Source: CAD feature listing. Evaluate the final solid. Frame: model axes, mm. Face numbers are marked on the shaded views. A direction names the side the tool comes from. Give positions to 0.01 mm unless a question says otherwise; leave off trailing zeros. Loops run counter-clockwise (first coordinate to the right, second up) from the corner with the lowest first, then second, coordinate; pieces in that order, holes last. Notation, with made-up numbers: (79, 1) -> (126, 1) arc R29 ccw to (126, 24) -> close; hole circle Ø2 at (33, 26.25). An arc over 180 degrees is marked (long way). Return JSON: item names as keys, results as strings. Group by question number.
(1) Pin query (flat end, axial travel): pin 1 (4 mm diameter, centred on x = 22.5, y = 47.5, fed in from -Z); pin 2 (3.5 mm diameter, centred on x = 8.5, y = -31.5, fed in from -Z); pin 3 (3 mm diameter, centred on y = 15.5, z = 10.5, fed in from +X); pin 4 (1.5 mm diameter, centred on x = -17, z = 6, fed in from +Y). Return the tip coordinate at first contact, or that it passes through.
(2) Ray query, line 1 (X direction, y = -28, z = 16.5); line 2 (Y direction, x = 0, z = 6.25); line 3 (Y direction, x = 12, z = 17.75). Return the intervals inside material, ascending. Write a range as from..to.
(3) Access query for the marked faces 1, 2 and 3. Directions: +Z, -Z, +X, -X, +Y, -Y. A direction counts if a zero-diameter tool reaches every point of the face in a straight line with its end or side. Return the directions, or none.
(4) Cut plane C-C on z = 6.5. Return loops of the section in (x, y).
(5) Draft query along Y for the marked faces 4, 5, 6 and 7. Return one class per face: released by +Y, released by -Y, zero draft, split by the parting line, or undercut.
(6) Cut plane B-B on y = 3.5. Return loops of the section in (x, z), then the cut area to 3 significant figures.
(7) Cut plane A-A on x = 0. Return loops of the section in (y, z).
(8) Cut plane D-D on x = -12. Give the number of separate pieces and of enclosed holes in the cut face, then the cut area to 3 significant figures.
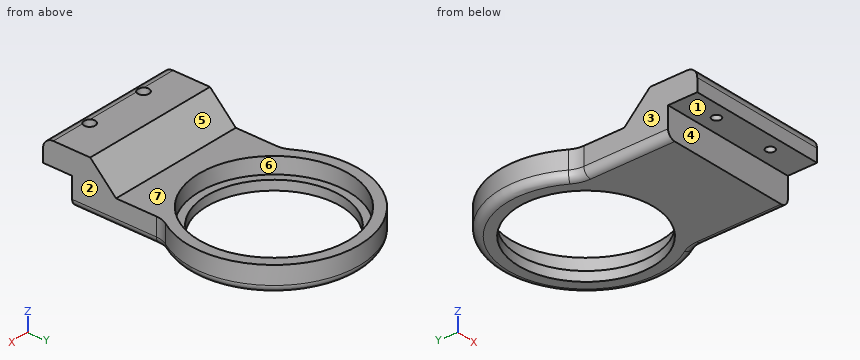
```python
from build123d import *

# Parameters (mm, degrees)
SKETCH_1_R          = 26
EXTRUDE_1_DEPTH     = 10
SKETCH_3_R          = 29
CUT_EXTRUDE_1_DEPTH = 6.3
FILLET_1_R          = 9
SKETCH_4_W          = 53.328443722
SKETCH_4_H          = 11.316007496
EXTRUDE_2_DEPTH     = 10
SKETCH_5_W          = 53.328443722
SKETCH_5_H          = 11.316007496
EXTRUDE_3_DEPTH     = 2
SKETCH_6_W          = 53.328443722
SKETCH_6_H          = 10
EXTRUDE_4_DEPTH     = 3
CHAMFER_1_SIZE      = 14
FILLET_3_R          = 3
SKETCH_7_R          = 1.7
CUT_EXTRUDE_2_DEPTH = 14
SKETCH_8_R          = 2.15
SKETCH_8_R_2        = 2.165
CUT_EXTRUDE_3_DEPTH = 6
SKETCH_9_W          = 53.328443722
SKETCH_9_H          = 11.316007496
CUT_EXTRUDE_4_DEPTH = 3
FILLET_4_R          = 4


with BuildPart() as part:
    # Sketch 1 → Extrude 1 (new body)
    with BuildSketch(Plane.XY):
        with BuildLine():
            Line((26.664221861, -27.841996252), (-26.664221861, -27.841996252))
            Line((-26.664221861, -27.841996252), (-26.664221861, 7.574088737))
            ThreePointArc((-26.664221861, 7.574088737), (0, 60.241390131), (26.664221861, 7.574088737))
            Line((26.664221861, 7.574088737), (26.664221861, -27.841996252))
        make_face()
        with Locations((0, 27.158003748)):
            Circle(SKETCH_1_R, mode=Mode.SUBTRACT)
    extrude(amount=EXTRUDE_1_DEPTH)

    # Sketch 3 → Cut-Extrude 1 (cut)
    with BuildSketch(Plane.XY.offset(10)):
        with Locations((0, 27.158003748)):
            Circle(SKETCH_3_R)
    extrude(amount=-CUT_EXTRUDE_1_DEPTH, mode=Mode.SUBTRACT)

    # Fillet 1
    fillet_1_edges = [part.edges().sort_by_distance(p)[0] for p in [
        (-26.664221861, 7.574088737, 5),
        (26.664221861, 7.574088737, 5),
    ]]
    fillet(fillet_1_edges, radius=FILLET_1_R)



with BuildPart() as body_2:
    # Sketch 4 → Extrude 2 (new body)
    with BuildSketch(Plane.XY.offset(10)):
        with Locations((0, -33.5)):
            Rectangle(SKETCH_4_W, SKETCH_4_H)
    extrude(amount=EXTRUDE_2_DEPTH)


with BuildPart() as part_1:
    add(part.part)

    add(body_2.part)  # Extrude 3 merges body 2
    # Sketch 5 → Extrude 3 (add)
    with BuildSketch(Plane(origin=(0, 0, 10), x_dir=(-1, 0, 0), z_dir=(0, 0, -1))):
        with Locations((0, -33.5)):
            Rectangle(SKETCH_5_W, SKETCH_5_H)
    extrude(amount=EXTRUDE_3_DEPTH)

    # Sketch 6 → Extrude 4 (add)
    with BuildSketch(Plane(origin=(0, -27.841996252, 0), x_dir=(1, 0, 0), z_dir=(0, 1, 0))):
        with Locations((0, -15)):
            Rectangle(SKETCH_6_W, SKETCH_6_H)
    extrude(amount=EXTRUDE_4_DEPTH)

    # Chamfer 1
    # the kernel refuses this chamfer: 14 mm, written as the material it adds along each edge
    with BuildSketch(Plane(origin=(-26.664221861, -24.841996252, 10), x_dir=(0, -0.027495876610586365, 0.9996219169112968), z_dir=(1, 0, 0))) as chamfer_1_piece_1_section:
        Polygon((CHAMFER_1_SIZE * 0.999621916911, -CHAMFER_1_SIZE * 0.0274958766106), (-CHAMFER_1_SIZE * 0.0274958766106, -CHAMFER_1_SIZE * 0.999621916911), (0, 0), align=None)
    chamfer_1_piece_1 = extrude(amount=53.328443723, mode=Mode.PRIVATE)
    chamfer_1_piece_1 = split(chamfer_1_piece_1, bisect_by=Plane(origin=(0, -19.845516644, 20), z_dir=(0, 0, -1)), keep=Keep.TOP, mode=Mode.PRIVATE)
    add(chamfer_1_piece_1)

    # Fillet 3
    fillet_3_edges = [part_1.edges().sort_by_distance(p)[0] for p in [
        (-26.664221861, -11.511986052, 0),
        (0, 60.241390131, 0),
        (-27.014230163, 7.303510743, 0),
        (27.014230163, 7.303510743, 0),
        (26.664221861, -11.511986052, 0),
    ]]
    fillet(fillet_3_edges, radius=FILLET_3_R)

    # Sketch 7 → Cut-Extrude 2 (cut)
    with BuildSketch(Plane(origin=(0, 0, 8), x_dir=(-1, 0, 0), z_dir=(0, 0, -1))):
        with Locations((-12, -33.841996252)):
            Circle(SKETCH_7_R)
        with Locations((12, -33.841996252)):
            Circle(SKETCH_7_R)
    extrude(amount=-CUT_EXTRUDE_2_DEPTH, mode=Mode.SUBTRACT)

    # Sketch 8 → Cut-Extrude 3 (cut)
    with BuildSketch(Plane.XY.offset(20)):
        with Locations((-12, -33.841996252)):
            Circle(SKETCH_8_R)
        with Locations((12, -33.841996252)):
            Circle(SKETCH_8_R_2)
    extrude(amount=-CUT_EXTRUDE_3_DEPTH, mode=Mode.SUBTRACT)

    # Sketch 9 → Cut-Extrude 4 (cut)
    with BuildSketch(Plane(origin=(0, 0, 8), x_dir=(-1, 0, 0), z_dir=(0, 0, -1))):
        with Locations((0, -33.5)):
            Rectangle(SKETCH_9_W, SKETCH_9_H)
    extrude(amount=-CUT_EXTRUDE_4_DEPTH, mode=Mode.SUBTRACT)

    # Fillet 4
    # the kernel refuses this fillet: 4 mm, written as the material it takes off along each edge
    with BuildSketch(Plane(origin=(36.664221861, -39.158003748, 20), x_dir=(0, 1, 0), z_dir=(-1, 0, 0))) as fillet_4_piece_1:
        with BuildLine():
            CenterArc((FILLET_4_R, FILLET_4_R), FILLET_4_R, 180, 90)
            Line((0, FILLET_4_R), (0, 0))
            Line((0, 0), (FILLET_4_R, 0))
        make_face()
    extrude(amount=73.328443723, mode=Mode.SUBTRACT)


solid = part_1.part
```
Answers:
{
 "1": {"pin 1": "z = 0", "pin 2": "z = 11", "pin 3": "x = 31.46", "pin 4": "y = 55.98"},
 "2": {"line 1": "-26.66..26.66", "line 2": "-27.84..-1.84, 56.16..60.24", "line 3": "-38.75..-36.01, -31.68..-18.59"},
 "3": {"face 1": "-Z, +X, -X, -Y", "face 2": "+Z, -Z, +X, -Y", "face 3": "+Z, -Z, -X, -Y"},
 "4": {"outline": "(-28.04, 9.6) arc R9 cw to (-26.66, 4.82) -> (-26.66, -27.84) -> (26.66, -27.84) -> (26.66, 4.82) arc R9 cw to (28.04, 9.6) arc R33.08 ccw (long way) to start; hole circle Ø58 at (0, 27.16)"},
 "5": {"face 4": "released by -Y", "face 5": "released by +Y", "face 6": "undercut", "face 7": "zero draft"},
 "6": {"outline": "(-26.66, 3) arc R3 ccw to (-23.66, 0) -> (-10.78, 0) -> (-10.78, 3.7) -> (-16.77, 3.7) -> (-16.77, 10) -> (-26.66, 10) -> close; (10.78, 0) -> (23.66, 0) arc R3 ccw to (26.66, 3) -> (26.66, 10) -> (16.77, 10) -> (16.77, 3.7) -> (10.78, 3.7) -> close", "area": "238 mm²"},
 "7": {"outline": "(-39.16, 11) -> (-27.84, 11) -> (-27.84, 0) -> (1.16, 0) -> (1.16, 3.7) -> (-1.84, 3.7) -> (-1.84, 10) -> (-10.84, 10) -> (-20.84, 20) -> (-35.16, 20) arc R4 ccw to (-39.16, 16) -> close; (53.16, 0) -> (57.24, 0) arc R3 ccw to (60.24, 3) -> (60.24, 10) -> (56.16, 10) -> (56.16, 3.7) -> (53.16, 3.7) -> close"},
 "8": {"separate pieces": "3", "enclosed holes": "0", "area": "535 mm²"}
}
